Part model, mm, in its own coordinate system. Face numbers are marked on the shaded views. Round coordinates to 2 decimals unless told otherwise and drop trailing zeros. One line per question, with ' | ' between items. Start each with the question number.
1) Mould opens along Z. For the marked faces 1, 2 and 3 say: pulls with the +Z half, pulls with the -Z half, needs draft (parallel to the pull), parting line crosses it, or undercut.
2) Drop flat-ended pins along their axis: pin 1 Ø1 at (y, z) = (-46.5, 10.5) entering from -X; pin 2 Ø1 at (x, y) = (-23.5, -25) entering from -Z; pin 3 Ø6 at (y, z) = (-50, 35) entering from +X. Give the stop position or say it passes through.
3) Wall check: probe 1 along Y at (x, z) = (-24, 0); probe 2 along Z at (x, y) = (-37.25, 0). Give the ranges that are in metal, low to high. Write a range as [from, to].
```python
from build123d import *


with BuildPart() as part:
    # Croquis1 → Revolución3 (revolve)
    with BuildSketch(Plane.XY):
        Polygon((-15.224198293, 10.01641294), (-35.224198293, 10.01641294), (-35.224198293, 20.01641294), (-30.224198293, 20.01641294), (-30.224198293, 80.01641294), (-50.224198293, 80.01641294), (-50.224198293, 100.01641294), (-45.224198293, 100.01641294), (-42.724198293, 90.01641294), (-40.224198293, 100.01641294), (-30.224198293, 100.01641294), (-27.724198293, 90.01641294), (-25.224198293, 100.01641294), (-20.224198293, 100.01641294), (-20.224198293, 80.01641294), (-20.224198293, 20.01641294), (-15.224198293, 20.01641294), align=None)
    revolve(axis=Axis((68.905582562, 0, 0), (-1, 0, 0)))


solid = part.part
```
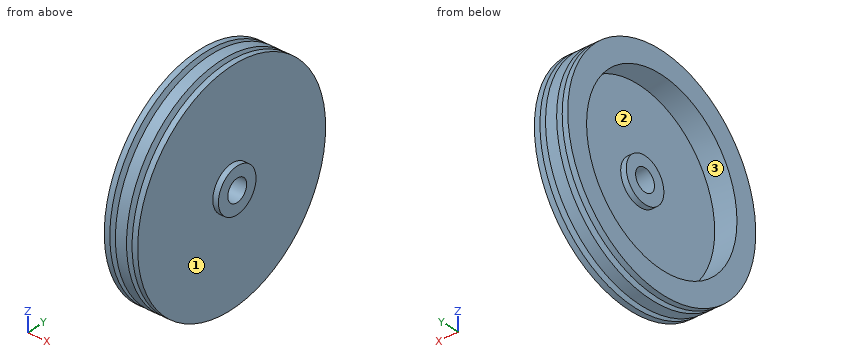
Answer key:
1) face 1: needs draft | face 2: undercut | face 3: undercut
2) pin 1: stops at x = -30.22 | pin 2: stops at z = -96.97 | pin 3: stops at x = -20.22
3) probe 1: y = [-100.02, -10.02], [10.02, 100.02] | probe 2: z = [-100.02, -80.02], [80.02, 100.02]
